Read the model definition and answer for the solid it produces. Units are mm, in the model's axes. Face numbers are marked on the shaded views. A direction names the side the tool comes from. Give positions to 0.01 mm unless a question says otherwise; leave off trailing zeros. Order: outer loops, then holes, each group sorted by start corner. A loop starts at its lowest first (then second) coordinate and runs counter-clockwise, first axis right, second up.
```python
from build123d import *

# Parameters (mm, degrees)
SKETCH_1_R      = 5
SKETCH_1_R_2    = 3
EXTRUDE_1_DEPTH = 5
SKETCH_2_R      = 8
SKETCH_2_R_2    = 5
EXTRUDE_2_DEPTH = 2
FILLET_1_R      = 0.2


with BuildPart() as part:
    # 草图1 → 凸台-拉伸1 (new, symmetric)
    with BuildSketch(Plane(origin=(0, 0, 0), x_dir=(1, 0, 0), z_dir=(0, 1, 0))):
        with Locations(Location((0, 0, 0), (0, 0, 270))):
            Circle(SKETCH_1_R)
        with Locations(Location((0, 0, 0), (0, 0, 270))):
            Circle(SKETCH_1_R_2, mode=Mode.SUBTRACT)
    extrude(amount=EXTRUDE_1_DEPTH, both=True)


with BuildPart() as body_2:
    # 草图2 → 凸台-拉伸2 (new body)
    with BuildSketch(Plane.XZ.offset(5)):
        with Locations(Location((0, 0, 0), (0, 0, 270))):
            Circle(SKETCH_2_R)
        with Locations(Location((0, 0, 0), (0, 0, 90))):
            Circle(SKETCH_2_R_2, mode=Mode.SUBTRACT)
    extrude(amount=-EXTRUDE_2_DEPTH)

    # Combine 1: union part
    add(part.part)

    # 圆角1
    fillet_1_edges = [body_2.edges().sort_by_distance(p)[0] for p in [
        (0, 5, -5),
        (0, -5, 8),
        (0, -3, 8),
    ]]
    fillet(fillet_1_edges, radius=FILLET_1_R)


solid = body_2.part
```
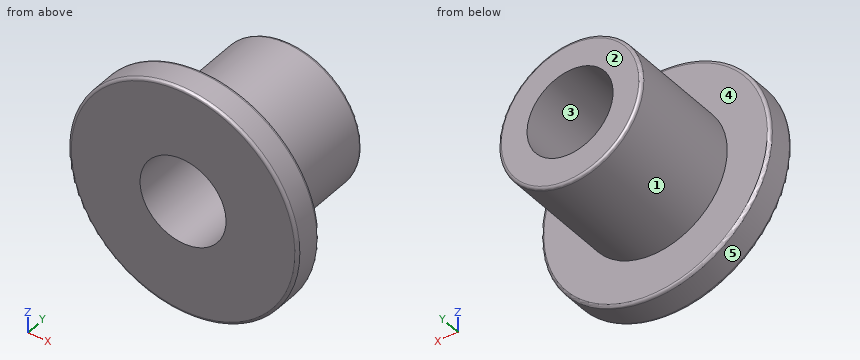
1) Given pin 1 (2 mm diameter, centred on y = -1.5, z = 4, fed in from -X); pin 2 (6 mm diameter, centred on y = -1, z = -2.5, fed in from -X); pin 3 (1 mm diameter, centred on x = -0.5, y = 2, fed in from -Z); pin 4 (6 mm diameter, centred on x = -1, z = 5.5, fed in from +Y), each flat-ended and moving along its own axis, determine where each tip first touches the part or whether it passes through.
Final values:
pin 1: stops at x = -4
pin 2: stops at x = -7.99
pin 3: stops at z = -5
pin 4: stops at y = 5
2) The part is cut by section B-B on x = 0. Determine the outline of the cut face in (y, z), and give its area (3 significant figures).
Final values:
outline: (-5, -7.8) arc R0.2 ccw to (-4.8, -8) - (-3.2, -8) arc R0.2 ccw to (-3, -7.8) - (-3, -5) - (4.8, -5) arc R0.2 ccw to (5, -4.8) - (5, -3) - (-5, -3) - close; (-5, 3) - (5, 3) - (5, 4.8) arc R0.2 ccw to (4.8, 5) - (-3, 5) - (-3, 7.8) arc R0.2 ccw to (-3.2, 8) - (-4.8, 8) arc R0.2 ccw to (-5, 7.8) - close
area: 51.9 mm2
3) A tool of negligible diameter and unlimited length cuts with its end or side. For the marked faces 1 and 2, from which of +Z, -Z, +X, -X, +Y, -Y can it reach the whole face along a straight path? Write none if from no direction.
Final values:
face 1: +Y
face 2: +Z, -Z, +X, -X, +Y
4) Consider L1, parallel to X at y = 2.25, z = 0; L2, parallel to Y at x = 5.5, z = 2.75; L3, parallel to X at y = 0.5, z = -4. Determine where each line is inside the solid, lowest interval first.
Final values:
L1: x = -5 to -3, 3 to 5
L2: y = -5 to -3
L3: x = -3 to 3
5) The part is cut by section A-A on z = 0. Determine the outline of the cut face in (x, y).
Final values:
outline: (-8, -4.8) arc R0.2 ccw to (-7.8, -5) - (-3, -5) - (-3, 5) - (-4.8, 5) arc R0.2 ccw to (-5, 4.8) - (-5, -3) - (-7.8, -3) arc R0.2 ccw to (-8, -3.2) - close; (3, -5) - (7.8, -5) arc R0.2 ccw to (8, -4.8) - (8, -3.2) arc R0.2 ccw to (7.8, -3) - (5, -3) - (5, 4.8) arc R0.2 ccw to (4.8, 5) - (3, 5) - close
6) For a pull along X with two mould halves and no side action, classify the marked faces 3, 4 and 5 as released by +X, released by -X, zero draft, split by the parting line, or undercut.
Final values:
face 3: undercut
face 4: zero draft
face 5: split by the parting line
7) The part is cut by section C-C on y = 1.5. Determine the outline of the cut face in (x, z).
Final values:
outline: circle Ø10 at (0, 0); hole circle Ø6 at (0, 0)
